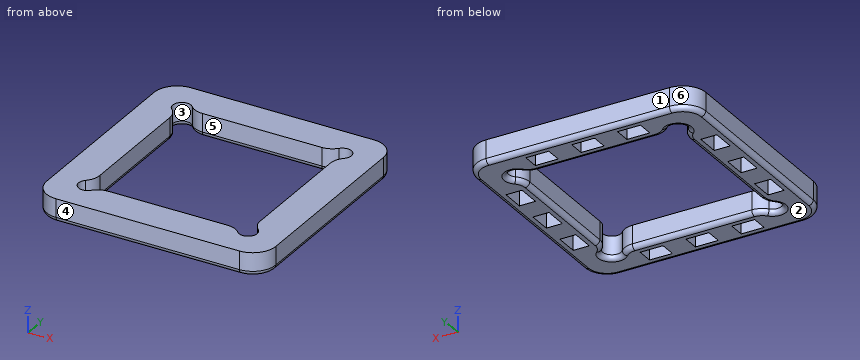
from build123d import *

# Parameters (mm, degrees)
CROQUIS1_W              = 100
CROQUIS1_H              = 100
SALIENTE_EXTRUIR1_DEPTH = 10
REDONDEO1_R             = 8
REDONDEO2_R             = 10
REDONDEO3_R             = 2
CROQUIS2_W              = 10
CROQUIS2_H              = 7
CROQUIS2_W_2            = 7
CROQUIS2_H_2            = 10
CORTAR_EXTRUIR1_DEPTH   = 7


with BuildPart() as part:
    # Croquis1 → Saliente-Extruir1 (new body)
    with BuildSketch(Plane.XY):
        with Locations((50, 50)):
            Rectangle(CROQUIS1_W, CROQUIS1_H)
        with BuildLine():
            Line((19, 15), (81, 15))
            ThreePointArc((81, 15), (87.828427125, 12.171572875), (85, 19))
            Line((85, 19), (85, 81))
            ThreePointArc((85, 81), (87.828427125, 87.828427125), (81, 85))
            Line((81, 85), (19, 85))
            ThreePointArc((19, 85), (12.171572875, 87.828427125), (15, 81))
            Line((15, 81), (15, 19))
            ThreePointArc((15, 19), (12.171572875, 12.171572875), (19, 15))
        make_face(mode=Mode.SUBTRACT)
    extrude(amount=SALIENTE_EXTRUIR1_DEPTH)

    # Redondeo1
    redondeo1_edges = [part.edges().sort_by_distance(p)[0] for p in [
        (15, 19, 5),
        (19, 15, 5),
        (81, 15, 5),
        (85, 19, 5),
        (85, 81, 5),
        (81, 85, 5),
        (19, 85, 5),
        (15, 81, 5),
    ]]
    fillet(redondeo1_edges, radius=REDONDEO1_R)

    # Redondeo2
    redondeo2_edges = [part.edges().sort_by_distance(p)[0] for p in [
        (0, 100, 5),
        (100, 100, 5),
        (100, 0, 5),
        (0, 0, 5),
    ]]
    fillet(redondeo2_edges, radius=REDONDEO2_R)

    # Redondeo3
    redondeo3_edges = [part.edges().sort_by_distance(p)[0] for p in [
        (87.828427125, 12.171572875, 0),
        (15, 50, 0),
        (12.171572875, 12.171572875, 0),
        (50, 15, 0),
        (85, 50, 0),
        (87.828427125, 87.828427125, 0),
        (50, 85, 0),
        (12.171572875, 87.828427125, 0),
        (85.697032567, 79.321714414, 0),
        (79.321714414, 85.697032567, 0),
        (20.678285586, 85.697032567, 0),
        (14.302967433, 79.321714414, 0),
        (20.678285586, 14.302967433, 0),
        (14.302967433, 20.678285586, 0),
        (79.321714414, 14.302967433, 0),
        (85.697032567, 20.678285586, 0),
        (50, 100, 0),
        (0, 50, 0),
        (100, 50, 0),
        (50, 0, 0),
        (97.071067812, 2.928932188, 0),
        (2.928932188, 2.928932188, 0),
        (2.928932188, 97.071067812, 0),
        (97.071067812, 97.071067812, 0),
    ]]
    fillet(redondeo3_edges, radius=REDONDEO3_R)

    # Croquis2 → Cortar-Extruir1 (cut)
    with BuildSketch(Plane(origin=(0, 0, 0), x_dir=(-1, 0, 0), z_dir=(0, 0, -1))):
        with Locations((-30, 7.5)):
            Rectangle(CROQUIS2_W, CROQUIS2_H)
        with Locations((-50, 7.5)):
            Rectangle(CROQUIS2_W, CROQUIS2_H)
        with Locations((-70, 7.5)):
            Rectangle(CROQUIS2_W, CROQUIS2_H)
        with Locations((-92.5, 30)):
            Rectangle(CROQUIS2_W_2, CROQUIS2_H_2)
        with Locations((-92.5, 50)):
            Rectangle(CROQUIS2_W_2, CROQUIS2_H_2)
        with Locations((-92.5, 70)):
            Rectangle(CROQUIS2_W_2, CROQUIS2_H_2)
        with Locations((-7.5, 30)):
            Rectangle(CROQUIS2_W_2, CROQUIS2_H_2)
        with Locations((-7.5, 50)):
            Rectangle(CROQUIS2_W_2, CROQUIS2_H_2)
        with Locations((-7.5, 70)):
            Rectangle(CROQUIS2_W_2, CROQUIS2_H_2)
        with Locations((-30, 92.5)):
            Rectangle(CROQUIS2_W, CROQUIS2_H)
        with Locations((-50, 92.5)):
            Rectangle(CROQUIS2_W, CROQUIS2_H)
        with Locations((-70, 92.5)):
            Rectangle(CROQUIS2_W, CROQUIS2_H)
    extrude(amount=-CORTAR_EXTRUIR1_DEPTH, mode=Mode.SUBTRACT)


solid = part.part
For this review, take the finished solid that the model builds, in its own axes (mm). Face numbers are marked on the shaded views. A direction names the side the tool comes from. Give positions to 0.01 mm unless a question says otherwise; leave off trailing zeros. Loops run counter-clockwise (first coordinate to the right, second up) from the corner with the lowest first, then second, coordinate; pieces in that order, holes last. Notation, with made-up numbers: M 17,63.25 L 54,63.25 A10 ccw 54,78.25 Z; hole C -9.5,-36 d8. An arc over 180 degrees is marked long. Answer as a JSON object with one key per item and string values. Group by question number.
Q1. For probe 1 along X at (y, z) = (32, 5.5); probe 2 along Y at (x, z) = (50, 0.5), list the stretches that pass through material, from the lowest coordinate up. Write a range as [from, to].
Q2. Add section B-B on z = 8.5. Give the boundary of the cut face in (x, y), and give its area (3 significant figures).
Q3. Mouldability with a two-part tool opening along Y and no side actions: class the marked faces 1, 2, 3 and 4 as +Y half, -Y half, draft (parallel to the pull), parting line (faces both ways), or undercut.
Q4. Add section D-D on y = 30. Give the boundary of the cut face in (x, z), and give its area (3 significant figures).
Q5. Tool access review of the marked faces 5 and 6: name each direction out of +Z, -Z, +X, -X, +Y, -Y from which nothing blocks a thin tool from reaching the whole face with its end or side.
Q6. Insertion check: P1, Ø10, axis at x = 20.5, y = 60, coming from the -Z side; P2, Ø3.5, axis at x = 67.5, y = 93, coming from the -Z side. Each pin has a flat end and moves straight along its axis. Give the tip position at first contact, or say it passes through.
Q7. Add section A-A on x = 61. Give the boundary of the cut face in (y, z).
Checked values:
{
 "1": {"probe 1": "[0, 4], [11, 15], [85, 89], [96, 100]", "probe 2": "[0.68, 4], [11, 14.32], [85.68, 89], [96, 99.32]"},
 "2": {"outline": "M 0,10 A10 ccw 10,0 L 90,0 A10 ccw 100,10 L 100,90 A10 ccw 90,100 L 10,100 A10 ccw 0,90 Z; hole M 12.33,17.98 A4 ccw long 17.98,12.33 A8 cw 23.94,15 L 76.06,15 A8 cw 82.02,12.33 A4 ccw long 87.67,17.98 A8 cw 85,23.94 L 85,76.06 A8 cw 87.67,82.02 A4 ccw long 82.02,87.67 A8 cw 76.06,85 L 23.94,85 A8 cw 17.98,87.67 A4 ccw long 12.33,82.02 A8 cw 15,76.06 L 15,23.94 A8 cw Z", "area": "4,840 mm²"},
 "3": {"face 1": "+Y half", "face 2": "draft", "face 3": "undercut", "face 4": "-Y half"},
 "4": {"outline": "M 0,2 A2 ccw 2,0 L 4,0 L 4,7 L 11,7 L 11,0 L 13,0 A2 ccw 15,2 L 15,10 L 0,10 Z; M 85,2 A2 ccw 87,0 L 89,0 L 89,7 L 96,7 L 96,0 L 98,0 A2 ccw 100,2 L 100,10 L 85,10 Z", "area": "199 mm²"},
 "5": {"face 5": "+Z, -Z", "face 6": "+Z, -Z, -X, +Y"},
 "6": {"P1": "through", "P2": "z = 7"},
 "7": {"outline": "M 0,2 A2 ccw 2,0 L 13,0 A2 ccw 15,2 L 15,10 L 0,10 Z; M 85,2 A2 ccw 87,0 L 98,0 A2 ccw 100,2 L 100,10 L 85,10 Z"}
}
